Verification items for the finished model (mm, model axes). A direction names the side the tool comes from. Round coordinates to 2 decimals unless told otherwise and drop trailing zeros. Write each loop counter-clockwise with the first axis right and the second up, starting at its lowest first coordinate (ties: lowest second). Pieces come first, ordered by that corner, then holes. Notation, with made-up numbers: M -18,66.5 L -2,66.5 A26 ccw -2,87.5 Z; hole C 56,56 d2. An arc over 180 degrees is marked long. Write each question's results on one line, items separated by ' | '.
from build123d import *

# Parameters (mm, degrees)
F1_DEPTH = 60
F2_R     = 5
F3_R     = 10
F4_SIZE  = 1


with BuildPart() as f1:
    # F0 (on Front) → F1 (new body)
    with BuildSketch(Plane.XZ):
        Polygon((-45.242744, -36.905519), (-45.242744, 63.094481), (-50.242744, 63.094481), (-50.242744, -41.905519), (49.757256, -41.905519), (49.757256, -86.905519), (54.757256, -86.905519), (54.757256, -36.905519), align=None)
    extrude(amount=F1_DEPTH)

    # F2
    f2_edges = [f1.edges().sort_by_distance(p)[0] for p in [
        (-45.242744, -30, -36.905519),
        (49.757256, -30, -41.905519),
    ]]
    fillet(f2_edges, radius=F2_R)

    # F3
    f3_edges = [f1.edges().sort_by_distance(p)[0] for p in [
        (54.757256, -30, -36.905519),
        (-50.242744, -30, -41.905519),
    ]]
    fillet(f3_edges, radius=F3_R)

    # F4
    f4_edges = [f1.edges().sort_by_distance(p)[0] for p in [
        (-45.242744, -30, 63.094481),
        (-50.242744, -30, 63.094481),
        (54.757256, -30, -86.905519),
        (49.757256, -30, -86.905519),
    ]]
    chamfer(f4_edges, length=F4_SIZE)


solid = f1.part
1) Sectioned sample at A-A, the plane y = -48. Record the cut outline in (x, z), and give its area (3 significant figures).
Calculated:
outline: M -50.24,-31.91 A10 ccw -40.24,-41.91 L 44.76,-41.91 A5 cw 49.76,-46.91 L 49.76,-85.91 L 50.76,-86.91 L 53.76,-86.91 L 54.76,-85.91 L 54.76,-46.91 A10 ccw 44.76,-36.91 L -40.24,-36.91 A5 cw -45.24,-31.91 L -45.24,62.09 L -46.24,63.09 L -49.24,63.09 L -50.24,62.09 Z | area: 1,220 mm²
2) Sectioned sample at C-C, the plane z = -14. Record the cut outline in (x, y).
Calculated:
outline: M -50.24,-60 L -45.24,-60 L -45.24,0 L -50.24,0 Z
3) Material ranges on line 1 (Z direction, x = -38, y = -30); line 2 (X direction, y = -32, z = -11); line 3 (X direction, y = -10, z = -34), recorded low to high. Write a range as [from, to].
Calculated:
line 1: z = [-41.91, -36.91] | line 2: x = [-50.24, -45.24] | line 3: x = [-50.02, -44.78]
4) Sectioned sample at B-B, the plane x = 14.5. Record the cut outline in (y, z).
Calculated:
outline: M -60,-41.91 L 0,-41.91 L 0,-36.91 L -60,-36.91 Z
5) Access from +Z, -Z, +X, -X, +Y, -Y to the whole of each face (thin tool, end or side, straight path). Record for faces 1 (the flat face through (2, -30, -41.906)), 2 (the flat face through (52, -30, -86.906)), 3 (the flat face through (-45.243, -30, 14)).
Calculated:
face 1: -Z, -X, +Y, -Y | face 2: -Z, +X, -X, +Y, -Y | face 3: +Z, +X, +Y, -Y
6) Depth check by flat-ended pin: P1, Ø8, axis at x = 6.5, y = -31, coming from the -Z side; P2, Ø8, axis at x = -15, y = -35.5, coming from the +Z side; P3, Ø8, axis at y = -17, z = -57.5, coming from the -X side. Enter the tip coordinate at first touch or a pass-through.
Calculated:
P1: stops at z = -41.91 | P2: stops at z = -36.91 | P3: stops at x = 49.76
